```python
from build123d import *

# Parameters (mm, degrees)
ESQUISSE1_W              = 35.68
ESQUISSE1_H              = 21.82
BOSS_EXTRU_1_DEPTH       = 6
ESQUISSE2_W              = 33.68
ESQUISSE2_H              = 19.82
ENL_V_MAT_EXTRU_1_DEPTH  = 5
ESQUISSE3_W              = 32.68
ESQUISSE3_H              = 18.82
ENL_V_MAT_EXTRU_2_DEPTH  = 43.120954405
ESQUISSE4_W              = 4
ESQUISSE4_H              = 16.82
ENL_V_MAT_EXTRU_3_DEPTH  = 5
ESQUISSE6_W              = 35.68
ESQUISSE6_H              = 8
BOSS_EXTRU_2_DEPTH       = 4
ESQUISSE7_W              = 35.68
ESQUISSE7_H              = 8
ENL_V_MAT_EXTRU_12_DEPTH = 2.5
CONG_2_R                 = 0.25
CONG_3_R                 = 2


with BuildPart() as part:
    # Esquisse1 → Boss.-Extru.1 (new body)
    with BuildSketch(Plane.XY):
        with Locations((17.84, 10.91)):
            Rectangle(ESQUISSE1_W, ESQUISSE1_H)
    extrude(amount=BOSS_EXTRU_1_DEPTH)

    # Esquisse2 → Enlèv. mat.-Extru.1 (cut)
    with BuildSketch(Plane.XY.offset(6)):
        with Locations((17.84, 10.91)):
            Rectangle(ESQUISSE2_W, ESQUISSE2_H)
    extrude(amount=-ENL_V_MAT_EXTRU_1_DEPTH, mode=Mode.SUBTRACT)

    # Esquisse3 → Enlèv. mat.-Extru.2 (cut, through all)
    with BuildSketch(Plane.XY.offset(1)):
        with Locations((17.84, 10.91)):
            Rectangle(ESQUISSE3_W, ESQUISSE3_H)
    extrude(amount=-ENL_V_MAT_EXTRU_2_DEPTH, mode=Mode.SUBTRACT)

    # Esquisse4 → Enlèv. mat.-Extru.3 (cut)
    with BuildSketch(Plane(origin=(35.68, 0, 0), x_dir=(0, 0, -1), z_dir=(1, 0, 0))):
        with Locations((-4, 10.41)):
            Rectangle(ESQUISSE4_W, ESQUISSE4_H)
    extrude(amount=-ENL_V_MAT_EXTRU_3_DEPTH, mode=Mode.SUBTRACT)

    # Esquisse6 → Boss.-Extru.2 (add)
    with BuildSketch(Plane.XY.offset(6)):
        with Locations((17.84, 25.82)):
            Rectangle(ESQUISSE6_W, ESQUISSE6_H)
    extrude(amount=-BOSS_EXTRU_2_DEPTH)

    # Esquisse7 → Enlèv. mat.-Extru.12 (cut)
    with BuildSketch(Plane.XY.offset(6)):
        with Locations((17.84, 25.82)):
            Rectangle(ESQUISSE7_W, ESQUISSE7_H)
    extrude(amount=-ENL_V_MAT_EXTRU_12_DEPTH, mode=Mode.SUBTRACT)

    # Congé2
    cong_2_edges = [part.edges().sort_by_distance(p)[0] for p in [
        (35.68, 1, 6),
        (1, 10.91, 6),
        (17.84, 1, 6),
        (34.68, 1.5, 6),
        (17.84, 20.82, 6),
        (34.68, 19.82, 6),
        (35.68, 20.32, 6),
        (35.18, 2, 6),
        (35.18, 18.82, 6),
        (17.84, 0, 6),
        (0, 10.91, 6),
        (17.84, 21.82, 6),
    ]]
    fillet(cong_2_edges, radius=CONG_2_R)

    # Congé3
    cong_3_edges = [part.edges().sort_by_distance(p)[0] for p in [
        (17.84, 21.82, 3.5),
    ]]
    fillet(cong_3_edges, radius=CONG_3_R)


solid = part.part
```
Could you check a few things on this model? Use its own coordinates, in mm. A direction names the side the tool comes from. Give positions to 0.01 mm unless a question says otherwise; leave off trailing zeros. Write each loop counter-clockwise with the first axis right and the second up, starting at its lowest first coordinate (ties: lowest second). Pieces come first, ordered by that corner, then holes. Notation, with made-up numbers: (23, 11) -> (64, 11) arc R25 ccw to (64, 46) -> close; hole circle Ø5 at (-12, 47.25). An arc over 180 degrees is marked (long way). Write each question's results on one line, items separated by ' | '.
1. Will these pins go through, and if not, where does the flat tip stop? pin 1 Ø6 at (x, y) = (21.5, 6.5) entering from +Z; pin 2 Ø5 at (x, y) = (27.5, 27) entering from +Z; pin 3 Ø1.1 at (x, y) = (35.5, 8) entering from +Z; pin 4 Ø1.4 at (y, z) = (14, 3) entering from -X.
Check sheet entries:
pin 1: passes through | pin 2: stops at z = 3.5 | pin 3: stops at z = 2 | pin 4: stops at x = 0
2. I need wall thicknesses on L1, parallel to X at y = 20.5, z = 3.55; L2, parallel to Y at x = 11.5, z = 1.75; L3, parallel to Y at x = 31, z = 3.1. Which ranges of each line are inside material? Lowest first, please.
Check sheet entries:
L1: x = 0 to 1, 34.68 to 35.68 | L2: y = 0 to 1, 20.82 to 21.82 | L3: y = 0 to 1, 20.82 to 29.82
3. On a 3-axis mill with a long thin cutter (end or side, diameter ignored), from which of +Z, -Z, +X, -X, +Y, -Y can I reach the whole of each face in a straight line? I mean faces 4 (the flat face through (1, 11, 3)), 5 (the flat face through (35, 2, 4)), 6 (the flat face through (18, 26, 2)), 7 (the flat face through (18, 29.82, 3)), 8 (the flat face through (17.6, 20.32, 0.5)). Say none if no direction works.
Check sheet entries:
face 4: +Z | face 5: +Z, +X | face 6: -Z, +X, -X, +Y | face 7: +Z, -Z, +X, -X, +Y | face 8: +Z, -Z
4. I want a section at D-D, the plane y = 4. Write out the boundary of the cut face in (x, z).
Check sheet entries:
outline: (0, 0) -> (1.5, 0) -> (1.5, 1) -> (1, 1) -> (1, 5.75) arc R0.25 ccw to (0.75, 6) -> (0.25, 6) arc R0.25 ccw to (0, 5.75) -> close; (34.18, 0) -> (35.68, 0) -> (35.68, 2) -> (34.68, 2) -> (34.68, 1) -> (34.18, 1) -> close
5. I want a section at A-A, the plane y = 19.5. Write out the boundary of the cut face in (x, z).
Check sheet entries:
outline: (0, 0) -> (1.5, 0) -> (1.5, 1) -> (1, 1) -> (1, 5.75) arc R0.25 ccw to (0.75, 6) -> (0.25, 6) arc R0.25 ccw to (0, 5.75) -> close; (34.18, 0) -> (35.68, 0) -> (35.68, 5.75) arc R0.25 ccw to (35.43, 6) -> (34.93, 6) arc R0.25 ccw to (34.68, 5.75) -> (34.68, 1) -> (34.18, 1) -> close
6. I want a section at C-C, the plane z = 4.65. Write out the boundary of the cut face in (x, y), then the cut area to 3 significant figures.
Check sheet entries:
outline: (0, 0) -> (35.68, 0) -> (35.68, 2) -> (34.68, 2) -> (34.68, 1) -> (1, 1) -> (1, 20.82) -> (34.68, 20.82) -> (34.68, 18.82) -> (35.68, 18.82) -> (35.68, 22.01) -> (0, 22.01) -> close | area: 101 mm²
7. If we mould it in two halves opening along X, with no side actions, what happens to faces 1 (the flat face through (34.18, 10.8, 0.5)), 2 (the flat face through (17.758, 21.225, 6)), 3 (the flat face through (35.68, 11.4, 1.6))? For each: released by +X, released by -X, zero draft, split by the parting line, or undercut.
Check sheet entries:
face 1: undercut | face 2: zero draft | face 3: released by +X
8. I want a section at B-B, the plane x = 7.5. Write out the boundary of the cut face in (y, z).
Check sheet entries:
outline: (0, 0) -> (1.5, 0) -> (1.5, 1) -> (1, 1) -> (1, 5.75) arc R0.25 ccw to (0.75, 6) -> (0.25, 6) arc R0.25 ccw to (0, 5.75) -> close; (20.32, 0) -> (21.82, 0) -> (21.82, 2) -> (29.82, 2) -> (29.82, 3.5) -> (23.82, 3.5) arc R2 cw to (21.82, 5.5) -> (21.82, 5.75) arc R0.25 ccw to (21.57, 6) -> (21.07, 6) arc R0.25 ccw to (20.82, 5.75) -> (20.82, 1) -> (20.32, 1) -> close
